Autodesk Inventor part; units mm, degrees
ref_plane "YZ Plane" through (0, 0, 0) normal (1, 0, 0) x (0, 1, 0)
ref_plane "XZ Plane" through (0, 0, 0) normal (0, 1, 0) x (-1, 0, 0)
ref_plane "XY Plane" through (0, 0, 0) normal (0, 0, 1) x (1, 0, 0)
sketch "Sketch1" plane through (0, 0, 0) normal (0, 1, 0) x (-1, 0, 0)
  line L0 (0, 0) -> (165.1, 0)
  line L1 (165.1, 0) -> (165.1, -203.2)
  line L2 (165.1, -203.2) -> (0, -203.2)
  line L3 (0, -203.2) -> (0, 0)
  line L4 (157.48, -195.58) -> (157.48, -7.62)
  line L5 (157.48, -7.62) -> (7.62, -7.62)
  line L6 (7.62, -7.62) -> (7.62, -195.58)
  line L7 (7.62, -195.58) -> (157.48, -195.58)
  circle A0 centre (82.55, -114.3) radius 31.75
  point P0 (82.55, -195.58)
  point P1 (157.48, -114.3)
  dimension "d0" = 203.2
  dimension "d1" = 165.1
  dimension "d2" = 7.62
  dimension "d3" = 63.5
  dimension "d4" = 88.9
extrude "Extrusion1" add sketch "Sketch1" along normal blind 6.35 contours L0 L1 L2 L3 | L7 L6 L5 L4 | A0
extrude "Extrusion2" add sketch "Sketch1" along normal blind 11.43 contours L7 L6 L5 L4
extrude "Extrusion3" cut sketch "Sketch1" along normal through all contours A0
properties part number "OGRobotRoof" material "ABS Plastic"
Geometry: final body of the model. Coordinates: model frame, mm. A direction names the side the tool comes from. Round coordinates to 2 decimals unless told otherwise and drop trailing zeros. Loops run counter-clockwise (first coordinate to the right, second up) from the corner with the lowest first, then second, coordinate; pieces in that order, holes last. Notation, with made-up numbers: (20, 27) -> (34, 27) arc R7 ccw to (34, 33) -> close; hole circle Ø1 at (72.5, 35). An arc over 180 degrees is marked (long way). Write each question's results on one line, items separated by ' | '.
Item 1: Cut plane D-D on z = -166.5. Return the cut outline in (x, y).
Answers below:
outline: (-165.1, 0) -> (0, 0) -> (0, 6.35) -> (-7.62, 6.35) -> (-7.62, 11.43) -> (-157.48, 11.43) -> (-157.48, 6.35) -> (-165.1, 6.35) -> close
Item 2: Pin query (flat end, axial travel): pin 1 Ø5.5 at (x, y) = (-73, 9.5) entering from +Z; pin 2 Ø2 at (y, z) = (7.5, -52) entering from -X; pin 3 Ø4 at (x, y) = (-63.5, 10) entering from -Z. Return the tip coordinate at first contact, or that it passes through.
Answers below:
pin 1: stops at z = -7.62 | pin 2: stops at x = -157.48 | pin 3: stops at z = -195.58
Item 3: Cut plane A-A on z = -114.3. Return the cut outline in (x, y), and give its area (3 significant figures).
Answers below:
outline: (-165.1, 0) -> (-114.3, 0) -> (-114.3, 11.43) -> (-157.48, 11.43) -> (-157.48, 6.35) -> (-165.1, 6.35) -> close; (-50.8, 0) -> (0, 0) -> (0, 6.35) -> (-7.62, 6.35) -> (-7.62, 11.43) -> (-50.8, 11.43) -> close | area: 1,080 mm²
Item 4: Pull-direction query (X, two-part tool) for faces 6 (the face through (-84, 3, -203.2)), 7 (the face through (-75.667, 5.635, -83.305)), 8 (the face through (-7.62, 9, -100)); classes: pulls with the +X half, pulls with the -X half, needs draft (parallel to the pull), parting line crosses it, or undercut.
Answers below:
face 6: needs draft | face 7: undercut | face 8: pulls with the +X half
Item 5: Line query: probe 1 along Z at (x, y) = (-82.55, 4.75); probe 2 along Z at (x, y) = (-82.55, 7.25); probe 3 along X at (y, z) = (10, -43). Output: solid intervals per line, ascending. Write a range as [from, to].
Answers below:
probe 1: z = [-203.2, -146.05], [-82.55, 0] | probe 2: z = [-195.58, -146.05], [-82.55, -7.62] | probe 3: x = [-157.48, -7.62]
Item 6: Set-up query: faces 1 (the face through (-165.1, 3, -100)), 2 (the face through (-82, 9, -195.58)), 3 (the face through (-81, 0, -78)), 4 (the face through (-157.48, 9, -103)), 5 (the face through (-84, 9, -7.62)). Return all of +Z, -Z, +X, -X, +Y, -Y with unobstructed straight access to the full face (end or side cutting, diameter ignored); none if empty.
Answers below:
face 1: +Z, -Z, -X, +Y, -Y | face 2: -Z, +X, -X, +Y | face 3: +Z, -Z, +X, -X, -Y | face 4: +Z, -Z, -X, +Y | face 5: +Z, +X, -X, +Y
Item 7: Cut plane C-C on x = -82.55. Return the cut outline in (y, z), and give its area (3 significant figures).
Answers below:
outline: (0, -203.2) -> (6.35, -203.2) -> (6.35, -195.58) -> (11.43, -195.58) -> (11.43, -146.05) -> (0, -146.05) -> close; (0, -82.55) -> (11.43, -82.55) -> (11.43, -7.62) -> (6.35, -7.62) -> (6.35, 0) -> (0, 0) -> close | area: 1,520 mm²
Item 8: Cut plane B-B on y = 8.25. Return the cut outline in (x, z).
Answers below:
outline: (-157.48, -195.58) -> (-7.62, -195.58) -> (-7.62, -7.62) -> (-157.48, -7.62) -> close; hole circle Ø63.5 at (-82.55, -114.3)
